The model under review builds one solid part; all positions refer to its coordinate system, in mm. A direction names the side the tool comes from. Give positions to 0.01 mm unless a question says otherwise; leave off trailing zeros. Loops run counter-clockwise (first coordinate to the right, second up) from the corner with the lowest first, then second, coordinate; pieces in that order, holes last. Notation, with made-up numbers: (45.25, -7) -> (73.25, -7) arc R14 cw to (73.25, 3) -> close; hole circle Ø11 at (59, 56). An arc over 180 degrees is marked (long way). Write each question's results on one line, items separated by ' | '. Start each with the question number.
Q1. Insertion check: pin 1 Ø6 at (y, z) = (191, -6) entering from -X; pin 2 Ø8 at (x, z) = (9, -9) entering from -Y; pin 3 Ø8 at (x, y) = (-5.5, 180.5) entering from +Z. Each pin has a flat end and moves straight along its axis. Give the tip position at first contact, or say it passes through.
Q2. We need section A-A (y = 60.5). Write out the cut boundary in (x, z), plus the area to 3 significant figures.
Q3. We need section B-B (y = 148). Write out the cut boundary in (x, z), plus the area to 3 significant figures.
Q4. Machinability: for faces 5 (the face through (12, 328, -11)), 6 (the face through (2, 137, -16)), 7 (the face through (-21, -15, -10)), which of the approach directions +Z, -Z, +X, -X, +Y, -Y give a long, thin tool a straight path to every point of the face, cutting with its end or side? Answer none if there is none.
Q5. Mouldability with a two-part tool opening along Y and no side actions: class faces 1 (the face through (7, 311, -11)), 2 (the face through (1, -15, -20)), 3 (the face through (-18, 2, -11)), 4 (the face through (-23, -15, -11)) as released by +Y, released by -Y, zero draft, split by the parting line, or undercut.
Q6. Wall thickness on L1, parallel to X at y = 312, z = -14; L2, parallel to X at y = 180.5, z = -20.9; L3, parallel to Y at x = -8, z = -7: over which ranges is each line inside the solid? List them lowest first. Write a range as [from, to].
from build123d import *

# Parameters (mm, degrees)
F1_DEPTH = 22
F3_DEPTH = 20
F5_DEPTH = 2
F6_DEPTH = 2
F7_DEPTH = 22
F9_DEPTH = 15


# Not quite as in the source:
# - a feature names something its author has since deleted; it is built from what else it names


with BuildPart() as f1:
    # F0 (on Top) → F1 (new body)
    with BuildSketch(Plane.XY):
        Polygon((-13, 345), (-13, 156.5), (-13, 2), (-23, 2), (-23, -32), (2, -32), (2, 311), (12, 311), (12, 345), align=None)
        Polygon((10, 313), (0, 313), (0, -30), (-21, -30), (-21, 0), (-11, 0), (-11, 156.5), (-11, 343), (10, 343), align=None, mode=Mode.SUBTRACT)
        Polygon((0, -30), (0, 313), (10, 313), (10, 343), (-11, 343), (-11, 156.5), (-11, 0), (-21, 0), (-21, -30), align=None)
        with BuildLine():
            ThreePointArc((-2.4999999702, 132.5), (-7.6213203138, 130.3786796564), (-5.4999999702, 135.5))
            ThreePointArc((-5.4999999702, 135.5), (-3.3786796266, 134.6213203436), (-2.4999999702, 132.5))
        make_face(mode=Mode.SUBTRACT)
        with BuildLine():
            ThreePointArc((-2.4999999702, 180.5), (-3.3786796266, 178.3786796564), (-5.4999999702, 177.5))
            ThreePointArc((-5.4999999702, 177.5), (-7.6213203138, 182.6213203436), (-2.4999999702, 180.5))
        make_face(mode=Mode.SUBTRACT)
    extrude(amount=-F1_DEPTH)

    # F0 (on Top) → F3 (cut)
    with BuildSketch(Plane.XY):
        Polygon((0, -30), (0, 313), (10, 313), (10, 343), (-11, 343), (-11, 156.5), (-11, 0), (-21, 0), (-21, -30), align=None)
        with BuildLine():
            ThreePointArc((-2.4999999702, 132.5), (-7.6213203138, 130.3786796564), (-5.4999999702, 135.5))
            ThreePointArc((-5.4999999702, 135.5), (-3.3786796266, 134.6213203436), (-2.4999999702, 132.5))
        make_face(mode=Mode.SUBTRACT)
        with BuildLine():
            ThreePointArc((-2.4999999702, 180.5), (-3.3786796266, 178.3786796564), (-5.4999999702, 177.5))
            ThreePointArc((-5.4999999702, 177.5), (-7.6213203138, 182.6213203436), (-2.4999999702, 180.5))
        make_face(mode=Mode.SUBTRACT)
    extrude(amount=-F3_DEPTH, mode=Mode.SUBTRACT)

    # F4 (on face) → F5 (cut)
    with BuildSketch(Plane.YZ.offset(2)):
        with BuildLine():
            Line((-0.1, 0), (-30.1, 0))
            Line((-30.1, 0), (-30.1, -5))
            ThreePointArc((-30.1, -5), (-15.1, -20), (-0.1, -5))
            Line((-0.1, -5), (-0.1, 0))
        make_face()
    extrude(amount=-F5_DEPTH, mode=Mode.SUBTRACT)

    # F2 (on face) → F6 (cut)
    with BuildSketch(Plane(origin=(-13, 0, 0), x_dir=(0, -1, 0), z_dir=(-1, 0, 0))):
        with BuildLine():
            Line((-343.0150201633, 0), (-343, -5))
            ThreePointArc((-343, -5), (-328.0000676811, -19.9549397135), (-313.0001353623, -5))
            Line((-313.0001353623, -5), (-313.0001353623, 0))
            Line((-313.0001353623, 0), (-343.0150201633, 0))
        make_face()
    extrude(amount=-F6_DEPTH, mode=Mode.SUBTRACT)

    # F0 (on Top) → F7 (cut)
    with BuildSketch(Plane.XY):
        with BuildLine():
            ThreePointArc((-2.4999999702, 180.5), (-7.6213203138, 182.6213203436), (-5.4999999702, 177.5))
            ThreePointArc((-5.4999999702, 177.5), (-3.3786796266, 178.3786796564), (-2.4999999702, 180.5))
        make_face()
    extrude(amount=-F7_DEPTH, mode=Mode.SUBTRACT)

    # F8 (on face) → F9 (cut)
    with BuildSketch(Plane(origin=(-13, 0, 0), x_dir=(0, -1, 0), z_dir=(-1, 0, 0))):
        with BuildLine():
            ThreePointArc((-191.5000676811, 0), (-156.5000676811, -18), (-121.5000676811, 0))
            Line((-121.5000676811, 0), (-156.5000676811, 0))
            Line((-156.5000676811, 0), (-191.5000676811, 0))
        make_face()
    extrude(amount=-F9_DEPTH, mode=Mode.SUBTRACT)


solid = f1.part
Output:
1) pin 1: x = -13 | pin 2: y = 311 | pin 3: z = -20
2) outline: (-13, -22) -> (2, -22) -> (2, 0) -> (0, 0) -> (0, -20) -> (-11, -20) -> (-11, 0) -> (-13, 0) -> close | area: 110 mm2
3) outline: (-13, -22) -> (2, -22) -> (2, -17.15) -> (0, -17.15) -> (0, -20) -> (-11, -20) -> (-11, -17.15) -> (-13, -17.15) -> close | area: 41.4 mm2
4) face 5: +Z, -Z, +X, +Y, -Y | face 6: +Z, -Z, +X, -Y | face 7: +Z
5) face 1: released by -Y | face 2: undercut | face 3: released by +Y | face 4: zero draft
6) L1: [-13, -11], [0, 12] | L2: [-13, -8.5], [-2.5, 2] | L3: [-32, -30], [343, 345]
